```python
from build123d import *

# Parameters (mm, degrees)
F0_W         = 79
F0_H         = 47
F0_W_2       = 77
F0_H_2       = 45
F1_DEPTH     = 17
F2_W         = 79
F2_H         = 47
F3_DEPTH     = 1
F4_W         = 2
F4_H         = 37
F5_DEPTH     = 79.001
F6_W         = 69
F6_H         = 2
F7_DEPTH     = 47.001
F8_R         = 1
F9_T1_DEPTH  = 19.5
F9_S5_W      = 1
F9_S5_H      = 1
F9_T6_DEPTH  = 1
F9_S11_W     = 1
F9_S11_H     = 1
F9_T12_DEPTH = 1
F9_S17_W     = 1
F9_S17_H     = 1
F9_T18_DEPTH = 1
F9_S23_W     = 1
F9_S23_H     = 1
F9_T24_DEPTH = 1


# Not quite as in the source:
# - a fillet or chamfer that OpenCascade refuses, or shapes differently, is made with other operations: its cross-section is extruded or revolved along the edge and cut away or added


with BuildPart() as f1:
    # F0 (on Front) → F1 (new body)
    with BuildSketch(Plane.XZ):
        with Locations((38.5, 22.5)):
            Rectangle(F0_W, F0_H)
        with Locations((38.5, 22.5)):
            Rectangle(F0_W_2, F0_H_2, mode=Mode.SUBTRACT)
    extrude(amount=F1_DEPTH)

    # F2 (on face) → F3 (join)
    with BuildSketch(Plane.XZ.offset(17)):
        with Locations((38.5, 22.5)):
            Rectangle(F2_W, F2_H)
    extrude(amount=F3_DEPTH)

    # F4 (on face) → F5 (cut, through all)
    with BuildSketch(Plane(origin=(-1, 0, 0), x_dir=(0, -1, 0), z_dir=(-1, 0, 0))):
        with Locations((1, 22.5)):
            Rectangle(F4_W, F4_H)
    extrude(amount=-F5_DEPTH, mode=Mode.SUBTRACT)

    # F6 (on face) → F7 (cut, through all)
    with BuildSketch(Plane(origin=(0, 0, -1), x_dir=(1, 0, 0), z_dir=(0, 0, -1))):
        with Locations((38.5, 1)):
            Rectangle(F6_W, F6_H)
    extrude(amount=-F7_DEPTH, mode=Mode.SUBTRACT)

    # F8
    f8_edges = [f1.edges().sort_by_distance(p)[0] for p in [
        (38.5, -18, 46),
        (-1, -18, 22.5),
        (38.5, -18, -1),
        (78, -18, 22.5),
    ]]
    fillet(f8_edges, radius=F8_R)

    # F9: fillet of radius 1 on 4 edges, made by hand

    # F9_s2 → F9_t1 (cut)
    with BuildSketch(Plane.XZ.offset(-2.5)):
        with BuildLine():
            ThreePointArc((-1, 45), (-0.7071067812, 45.7071067812), (0, 46))
            Line((0, 46), (-1, 46))
            Line((-1, 46), (-1, 45))
        make_face()
        with BuildLine():
            ThreePointArc((-1, 0), (-0.7071067812, -0.7071067812), (0, -1))
            Line((0, -1), (-1, -1))
            Line((-1, -1), (-1, 0))
        make_face()
        with BuildLine():
            ThreePointArc((77, -1), (77.7071067812, -0.7071067812), (78, 0))
            Line((78, 0), (78, -1))
            Line((78, -1), (77, -1))
        make_face()
        with BuildLine():
            ThreePointArc((77, 46), (77.7071067812, 45.7071067812), (78, 45))
            Line((78, 45), (78, 46))
            Line((78, 46), (77, 46))
        make_face()
    extrude(amount=F9_T1_DEPTH, mode=Mode.SUBTRACT)


with BuildPart() as f9_tool4:
    # F9_s5 → F9_t6 (new body)
    with BuildSketch(Plane.XY.offset(45)):
        with Locations((77.5, -17.5)):
            Rectangle(F9_S5_W, F9_S5_H)
    extrude(amount=F9_T6_DEPTH)

    # F9_s7 → F9_t8 (revolve, cut)
    with BuildSketch(Plane(origin=(77, -17, 45), x_dir=(-0.7071067812, 0.7071067812, 0), z_dir=(0.7071067812, 0.7071067812, 0))):
        with BuildLine():
            ThreePointArc((0, -1), (1, 0), (0, 1))
            Line((0, 1), (0, -1))
        make_face()
    revolve(axis=Axis((77, -17, 45), (0, 0, 1)), mode=Mode.SUBTRACT)


with BuildPart() as f1_1:
    add(f1.part)

    # F9_t3: cut F9_tool4
    add(f9_tool4.part, mode=Mode.SUBTRACT)


with BuildPart() as f9_tool10:
    # F9_s11 → F9_t12 (new body)
    with BuildSketch(Plane.XY):
        with Locations((77.5, -17.5)):
            Rectangle(F9_S11_W, F9_S11_H)
    extrude(amount=-F9_T12_DEPTH)

    # F9_s13 → F9_t14 (revolve, cut)
    with BuildSketch(Plane(origin=(77, -17, 0), x_dir=(-0.7071067812, 0.7071067812, 0), z_dir=(-0.7071067812, -0.7071067812, 0))):
        with BuildLine():
            ThreePointArc((0, -1), (1, 0), (0, 1))
            Line((0, 1), (0, -1))
        make_face()
    revolve(axis=Axis((77, -17, 0), (0, 0, -1)), mode=Mode.SUBTRACT)


with BuildPart() as f1_2:
    add(f1_1.part)

    # F9_t9: cut F9_tool10
    add(f9_tool10.part, mode=Mode.SUBTRACT)


with BuildPart() as f9_tool16:
    # F9_s17 → F9_t18 (new body)
    with BuildSketch(Plane.YZ):
        with Locations((-17.5, -0.5)):
            Rectangle(F9_S17_W, F9_S17_H)
    extrude(amount=-F9_T18_DEPTH)

    # F9_s19 → F9_t20 (revolve, cut)
    with BuildSketch(Plane(origin=(0, -17, 0), x_dir=(0, 0.7071067812, 0.7071067812), z_dir=(0, -0.7071067812, 0.7071067812))):
        with BuildLine():
            ThreePointArc((0, -1), (1, 0), (0, 1))
            Line((0, 1), (0, -1))
        make_face()
    revolve(axis=Axis((0, -17, 0), (-1, 0, 0)), mode=Mode.SUBTRACT)


with BuildPart() as f1_3:
    add(f1_2.part)

    # F9_t15: cut F9_tool16
    add(f9_tool16.part, mode=Mode.SUBTRACT)


with BuildPart() as f9_tool22:
    # F9_s23 → F9_t24 (new body)
    with BuildSketch(Plane.YZ):
        with Locations((-17.5, 45.5)):
            Rectangle(F9_S23_W, F9_S23_H)
    extrude(amount=-F9_T24_DEPTH)

    # F9_s25 → F9_t26 (revolve, cut)
    with BuildSketch(Plane(origin=(0, -17, 45), x_dir=(0, 0.7071067812, -0.7071067812), z_dir=(0, 0.7071067812, 0.7071067812))):
        with BuildLine():
            ThreePointArc((0, -1), (1, 0), (0, 1))
            Line((0, 1), (0, -1))
        make_face()
    revolve(axis=Axis((0, -17, 45), (-1, 0, 0)), mode=Mode.SUBTRACT)


with BuildPart() as f1_4:
    add(f1_3.part)

    # F9_t21: cut F9_tool22
    add(f9_tool22.part, mode=Mode.SUBTRACT)


solid = f1_4.part
```
Could you check a few things on this model? Use its own coordinates, in mm. A direction names the side the tool comes from. Coordinates: 2 decimals unless noted, no trailing zeros. Write each loop counter-clockwise with the first axis right and the second up, starting at its lowest first coordinate (ties: lowest second). Pieces come first, ordered by that corner, then holes. Notation, with made-up numbers: (-37.5, 46) -> (-17.5, 46) arc R18 cw to (-17.5, 57) -> close; hole circle Ø4 at (-14, -10.5). An arc over 180 degrees is marked (long way). Return JSON: item names as keys, results as strings.
(1) Imagine slicing it at C-C, the plane x = 72. Please give me the cut outline in (y, z).
Numbers:
{"outline": "(-18, 0) arc R1 ccw to (-17, -1) -> (-2, -1) -> (-2, 0) -> (-17, 0) -> (-17, 45) -> (-2, 45) -> (-2, 46) -> (-17, 46) arc R1 ccw to (-18, 45) -> close"}
(2) Imagine slicing it at A-A, the plane y = -7.75. Please give me the cut outline in (x, z), then the cut area to 3 significant figures.
Numbers:
{"outline": "(-1, 0) arc R1 ccw to (0, -1) -> (77, -1) arc R1 ccw to (78, 0) -> (78, 45) arc R1 ccw to (77, 46) -> (0, 46) arc R1 ccw to (-1, 45) -> close; hole (0, 0) -> (77, 0) -> (77, 45) -> (0, 45) -> close", "area": "247 mm2"}
(3) We'd pull the mould along X, two halves only. Please class faces 3 (the flat face through (78, -8, 22)), 4 (the flat face through (38, -18, 23)), 5 (the flat face through (77, -8, 22)): +X half, -X half, draft (parallel to the pull), parting line (faces both ways), or undercut.
Numbers:
{"face 3": "+X half", "face 4": "draft", "face 5": "undercut"}
(4) I need wall thicknesses on L1, parallel to X at y = -8.5, z = 10; L2, parallel to Z at x = 61, y = -2.5; L3, parallel to Y at x = 8.5, z = 23.5. Which ranges of each line are inside material? Lowest first, please.
Numbers:
{"L1": "x = -1 to 0, 77 to 78", "L2": "z = -1 to 0, 45 to 46", "L3": "y = -18 to -17"}
(5) Imagine slicing it at B-B, the plane z = 39. Please give me the cut outline in (x, y), then the cut area to 3 significant figures.
Numbers:
{"outline": "(-1, -17) arc R1 ccw to (0, -18) -> (77, -18) arc R1 ccw to (78, -17) -> (78, -2) -> (77, -2) -> (77, -17) -> (0, -17) -> (0, -2) -> (-1, -2) -> close", "area": "109 mm2"}
(6) Which directions (+Z, -Z, +X, -X, +Y, -Y) give clear straight access to the entire face, cutting with the end or side of a thin tool? Please do faces 1 (the flat face through (0, -8, 22)), 2 (the flat face through (77.13, 0, -0.13)).
Numbers:
{"face 1": "+Y", "face 2": "+Z, -Z, +X, -X, +Y"}
(7) I'm going to push flat-ended pins straight in: pin 1 (0.8 mm diameter, centred on x = 31.5, z = 45.5, fed in from +Y); pin 2 (1 mm diameter, centred on x = 36.5, z = 16.5, fed in from +Y); pin 3 (0.8 mm diameter, centred on y = -1, z = 45.5, fed in from -X) (3 decimals). Where does each tip first touch, or does it pass through?
Numbers:
{"pin 1": "stops at y = -2", "pin 2": "stops at y = -17", "pin 3": "stops at x = -0.995"}
